Geometry: final body of the model. Coordinates: model frame, mm. A direction names the side the tool comes from. Round coordinates to 2 decimals unless told otherwise and drop trailing zeros. Write each loop counter-clockwise with the first axis right and the second up, starting at its lowest first coordinate (ties: lowest second). Pieces come first, ordered by that corner, then holes. Notation, with made-up numbers: M -8,26.5 L 5,26.5 A27 cw 5,49.5 Z; hole C 28,42.25 d6. An arc over 180 degrees is marked long. Use one line per item in the form item = value. Start each with the question number.
Item 1: Reachability of faces 1 (the cylindrical face through (2.5, 22.3, -5)), 2 (the cylindrical face through (52.474, 2.465, -4.609)), 3 (the cylindrical face through (1.48, 16.14, -28.04)), 4 (the cylindrical face through (1.479, 6.95, -15.546)), 5 (the cylindrical face through (1.89, 19.63, -10.18)) from +Z, -Z, +X, -X, +Y, -Y: full face, straight path, thin tool, end or side. Return the list, or none.
Item 2: Section query A-A (x = 30.5). Return loops of the section in (y, z) (3 decimals).
Item 3: Section query B-B (z = -22.5). Return loops of the section in (x, y), and give its area (3 significant figures).
Item 4: Ray query, probe 1 along X at (y, z) = (0.95, -22.5); probe 2 along Y at (x, z) = (4.1, -16.5); probe 3 along X at (y, z) = (5.25, -23.5). Return the intervals inside material, ascending.
Item 5: Pull-direction query (X, two-part tool) for faces 6 (the cylindrical face through (4.014, 8.602, -15.026)), 7 (the flat face through (23, 9, -34)), 8 (the cylindrical face through (52.99, 6.63, -2.85)); classes: pulls with the +X half, pulls with the -X half, needs draft (parallel to the pull), parting line crosses it, or undercut.
Item 6: Pin query (flat end, axial travel): pin 1 Ø7 at (x, z) = (49.5, -5) entering from +Y; pin 2 Ø1.2 at (y, z) = (7.5, -28.5) entering from +X; pin 3 Ø4 at (x, z) = (49.5, -5) entering from -Y; pin 4 Ø5 at (x, z) = (8, -26) entering from -Y. Return the tip coordinate at first contact, or that it passes through.
Item 7: Section query C-C (y = 15.25). State how many separate pieces and enclosed holes the cut face has, and give its area (3 significant figures).
from build123d import *

# Parameters (mm, degrees)
BOSS_EXTRUDE1_DEPTH     = 22.5
CUT_EXTRUDE1_DEPTH      = 17.5
CUT_EXTRUDE2_DEPTH      = 15
CUT_EXTRUDE2_DEPTH_BACK = 66.29356783
SKETCH4_R               = 1
SKETCH5_W               = 10.5
SKETCH5_H               = 12.5
CUT_EXTRUDE3_DEPTH      = 20
SKETCH6_R               = 1.4
CUT_EXTRUDE4_DEPTH      = 10
SKETCH8_R               = 1
SKETCH8_W               = 24
SKETCH8_H               = 13
CUT_EXTRUDE6_DEPTH      = 68.810397433
SKETCH9_R               = 1.5
CUT_EXTRUDE7_DEPTH      = 70.269401614
SKETCH10_R              = 3
CUT_EXTRUDE8_DEPTH      = 5
SKETCH14_W              = 12
SKETCH14_H              = 17.5
BOSS_EXTRUDE3_DEPTH     = 3.5
SKETCH11_R              = 1.5
CUT_EXTRUDE9_DEPTH      = 10
SKETCH16_R              = 2
CUT_EXTRUDE11_DEPTH     = 2
SKETCH18_W              = 6.5
SKETCH18_H              = 2.5
CUT_EXTRUDE12_DEPTH     = 70.269401614
CUT_EXTRUDE14_DEPTH     = 70.269401614
SKETCH22_R              = 1.6
CUT_EXTRUDE15_DEPTH     = 70.269401614
SKETCH23_R              = 3
CUT_EXTRUDE18_DEPTH     = 3
CUT_EXTRUDE19_DEPTH     = 10
SKETCH25_W              = 6.5
SKETCH25_H              = 11.5
CUT_EXTRUDE20_DEPTH     = 2


with BuildPart() as part:
    # Sketch2 → Boss-Extrude1 (new body)
    with BuildSketch(Plane(origin=(0, 0, 0), x_dir=(1, 0, 0), z_dir=(0, 1, 0))):
        with BuildLine():
            Line((0, 0), (46, 0))
            ThreePointArc((46, 0), (53.071067812, 2.928932188), (56, 10))
            Line((56, 10), (56, 24))
            ThreePointArc((56, 24), (53.071067812, 31.071067812), (46, 34))
            Line((46, 34), (0, 34))
            Line((0, 34), (0, 14))
            Line((0, 14), (-6.5, 14))
            Line((-6.5, 14), (-6.5, 0))
            Line((-6.5, 0), (0, 0))
        make_face()
    extrude(amount=BOSS_EXTRUDE1_DEPTH)

    # Sketch3 → Cut-Extrude1 (cut)
    with BuildSketch(Plane(origin=(0, 22.5, 0), x_dir=(1, 0, 0), z_dir=(0, 1, 0))):
        with BuildLine():
            Line((45, 32), (5, 32))
            Line((5, 32), (5, 3.5))
            Line((5, 3.5), (17, 3.5))
            Line((17, 3.5), (17, 2))
            Line((17, 2), (45, 2))
            Line((45, 2), (45, 4))
            ThreePointArc((45, 4), (46.464466094, 7.535533906), (50, 9))
            Line((50, 9), (54, 9))
            Line((54, 9), (54, 25))
            Line((54, 25), (50, 25))
            ThreePointArc((50, 25), (46.464466094, 26.464466094), (45, 30))
            Line((45, 30), (45, 32))
        make_face()
    extrude(amount=-CUT_EXTRUDE1_DEPTH, mode=Mode.SUBTRACT)

    # Sketch4 → Cut-Extrude2 (cut, two sides: drawn at the far end of the back side and taken through both)
    with BuildSketch(Plane(origin=(5, 0, 0), x_dir=(0, 0, -1), z_dir=(1, 0, 0)).offset(-CUT_EXTRUDE2_DEPTH_BACK)):
        with Locations(Location((28.5, 15.25, 0), (0, 0, 180))):
            Circle(SKETCH4_R)
        with Locations(Location((28.5, 7.25, 0), (0, 0, 180))):
            Circle(SKETCH4_R)
        with Locations(Location((16.5, 7.25, 0), (0, 0, 180))):
            Circle(SKETCH4_R)
        with Locations(Location((16.5, 15.25, 0), (0, 0, 180))):
            Circle(SKETCH4_R)
    extrude(amount=CUT_EXTRUDE2_DEPTH + CUT_EXTRUDE2_DEPTH_BACK, mode=Mode.SUBTRACT)

    # Sketch5 → Cut-Extrude3 (cut)
    with BuildSketch(Plane.ZY.offset(6.5)):
        with Locations((-8.75, 11.5)):
            Rectangle(SKETCH5_W, SKETCH5_H)
    extrude(amount=-CUT_EXTRUDE3_DEPTH, mode=Mode.SUBTRACT)

    # Sketch6 → Cut-Extrude4 (cut)
    with BuildSketch(Plane(origin=(0, 22.5, 0), x_dir=(1, 0, 0), z_dir=(0, 1, 0))):
        with Locations(Location((0.5, 10, 0), (0, 0, 270))):
            Circle(SKETCH6_R)
    extrude(amount=-CUT_EXTRUDE4_DEPTH, mode=Mode.SUBTRACT)

    # Sketch8 → Cut-Extrude6 (cut, through all)
    with BuildSketch(Plane(origin=(0, 5, 0), x_dir=(1, 0, 0), z_dir=(0, 1, 0))):
        with Locations(Location((50.6, 17, 0), (0, 0, 270))):
            Circle(SKETCH8_R)
        with Locations(Location((22.4, 17, 0), (0, 0, 270))):
            Circle(SKETCH8_R)
        with Locations((36.5, 17)):
            Rectangle(SKETCH8_W, SKETCH8_H)
    extrude(amount=-CUT_EXTRUDE6_DEPTH, mode=Mode.SUBTRACT)

    # Sketch9 → Cut-Extrude7 (cut, through all)
    with BuildSketch(Plane(origin=(0, 22.5, 0), x_dir=(1, 0, 0), z_dir=(0, 1, 0))):
        with Locations(Location((49.5, 29, 0), (0, 0, 270))):
            Circle(SKETCH9_R)
        with Locations(Location((49.5, 5, 0), (0, 0, 270))):
            Circle(SKETCH9_R)
    extrude(amount=-CUT_EXTRUDE7_DEPTH, mode=Mode.SUBTRACT)

    # Sketch10 → Cut-Extrude8 (cut)
    with BuildSketch(Plane.XZ):
        with Locations(Location((49.5, -5, 0), (0, 0, 270))):
            Circle(SKETCH10_R)
        with Locations(Location((49.5, -29, 0), (0, 0, 270))):
            Circle(SKETCH10_R)
    extrude(amount=-CUT_EXTRUDE8_DEPTH, mode=Mode.SUBTRACT)

    # Sketch14 → Boss-Extrude3 (add, symmetric)
    with BuildSketch(Plane.XY.offset(-22.5)):
        with Locations((11, 13.75)):
            Rectangle(SKETCH14_W, SKETCH14_H)
    extrude(amount=BOSS_EXTRUDE3_DEPTH, both=True)

    # Sketch11 → Cut-Extrude9 (cut)
    with BuildSketch(Plane.XZ):
        with Locations(Location((8, -8, 0), (0, 0, 270))):
            Circle(SKETCH11_R)
        with Locations(Location((8, -26, 0), (0, 0, 270))):
            Circle(SKETCH11_R)
    extrude(amount=-CUT_EXTRUDE9_DEPTH, mode=Mode.SUBTRACT)

    # Sketch16 → Cut-Extrude11 (cut)
    with BuildSketch(Plane(origin=(5, 0, 0), x_dir=(0, 0, -1), z_dir=(1, 0, 0))):
        with Locations((28.5, 15.25)):
            Circle(SKETCH16_R)
        with Locations((28.5, 7.25)):
            Circle(SKETCH16_R)
        with Locations((16.5, 7.25)):
            Circle(SKETCH16_R)
        with Locations((16.5, 15.25)):
            Circle(SKETCH16_R)
    extrude(amount=-CUT_EXTRUDE11_DEPTH, mode=Mode.SUBTRACT)

    # Sketch18 → Cut-Extrude12 (cut, through all)
    with BuildSketch(Plane(origin=(0, 22.5, 0), x_dir=(1, 0, 0), z_dir=(0, 1, 0))):
        with Locations((-3.25, 1.25)):
            Rectangle(SKETCH18_W, SKETCH18_H)
    extrude(amount=-CUT_EXTRUDE12_DEPTH, mode=Mode.SUBTRACT)

    # Sketch21 → Cut-Extrude14 (cut, through all)
    with BuildSketch(Plane.XY):
        Polygon((5, 22.5), (56, 11.25), (56, 22.5), align=None)
    extrude(amount=-CUT_EXTRUDE14_DEPTH, mode=Mode.SUBTRACT)

    # Sketch22 → Cut-Extrude15 (cut, through all)
    with BuildSketch(Plane.XZ):
        with Locations(Location((14, -22.5, 0), (0, 0, 270))):
            Circle(SKETCH22_R)
    extrude(amount=-CUT_EXTRUDE15_DEPTH, mode=Mode.SUBTRACT)

    # Sketch23 → Cut-Extrude18 (cut)
    with BuildSketch(Plane.XZ):
        with Locations(Location((14, -22.5, 0), (0, 0, 270))):
            Circle(SKETCH23_R)
    extrude(amount=-CUT_EXTRUDE18_DEPTH, mode=Mode.SUBTRACT)

    # Sketch26 → Cut-Extrude19 (cut)
    with BuildSketch(Plane.ZY):
        with BuildLine():
            Line((-5.916515139, 22.5), (-4.083484861, 22.5))
            ThreePointArc((-4.083484861, 22.5), (-5, 22.3), (-5.916515139, 22.5))
        make_face()
    extrude(amount=-CUT_EXTRUDE19_DEPTH, mode=Mode.SUBTRACT)

    # Sketch25 → Cut-Extrude20 (cut)
    with BuildSketch(Plane(origin=(0, 22.5, 0), x_dir=(1, 0, 0), z_dir=(0, 1, 0))):
        with Locations((-3.25, 8.25)):
            Rectangle(SKETCH25_W, SKETCH25_H)
    extrude(amount=-CUT_EXTRUDE20_DEPTH, mode=Mode.SUBTRACT)


solid = part.part
Working result:
q1.face_1 = +X, -X, +Y
q1.face_2 = -Y
q1.face_3 = +X, -X
q1.face_4 = -X
q1.face_5 = +Y
q2.outline = M 0,-34 L 16.875,-34 L 16.875,-32 L 5,-32 L 5,-23.5 L 0,-23.5 Z; M 0,-10.5 L 5,-10.5 L 5,-2 L 16.875,-2 L 16.875,0 L 0,0 Z
q3.outline = M 0,0 L 11,0 L 11,3 L 12.4,3 L 12.4,20.87 L 5,22.5 L 0,22.5 Z; M 15.6,3 L 17,3 L 17,0 L 24.5,0 L 24.5,5 L 17,5 L 17,19.85 L 15.6,20.16 Z; M 48.5,0 L 56,0 L 56,11.25 L 54,11.69 L 54,5 L 48.5,5 Z
q3.area = 381 mm²
q4.probe_1 = 0 to 11, 17 to 24.5, 48.5 to 56
q4.probe_2 = 0 to 5.25, 9.25 to 13.25, 17.25 to 22.5
q4.probe_3 = 0 to 12.75, 15.25 to 17, 54 to 56
q5.face_6 = undercut
q5.face_7 = needs draft
q5.face_8 = pulls with the +X half
q6.pin_1 = 13.46
q6.pin_2 = 55.21
q6.pin_3 = 5
q6.pin_4 = 0
q7.separate_pieces = 4
q7.enclosed_holes = 1
q7.area = 321 mm²
